Drawing for the job (mm, zero at the part's lowest x, y, z). Coordinates: 2 decimals unless noted, no trailing zeros. Write each loop counter-clockwise with the first axis right and the second up, starting at its lowest first coordinate (ties: lowest second). Pieces come first, ordered by that corner, then holes. Notation, with made-up numbers: M 76.5,29.5 L 108.5,29.5 A17 ccw 108.5,51.5 Z; hole C 18,-19 d4. An arc over 180 degrees is marked long. Put each result on its own line as item: value. Start each with the question number.
Q1. Cut at B-B (z = 5). Write the cut outline in (x, y).
Q2. Cut at D-D (y = 2.75). Write the cut outline in (x, z) (1 decimal).
Q3. Cut at C-C (y = 11.5). Write the cut outline in (x, z).
Q4. Pull direction X, two halves, no side cores. Call the marked faces 1 and 2: pulls with the +X half, pulls with the -X half, needs draft (parallel to the pull), parting line crosses it, or undercut.
Q5. Drill centre lines: line 1 along Z through (x, y) = (8.5, 3.75); line 2 along Y through (x, z) = (7.5, 9) (1 decimal); line 3 along X through (y, z) = (10.25, 3.5). Where is each one in solid material? Low to high.
Q6. Cut at A-A (x = 5). Write the cut outline in (y, z).
Q7. Drop flat-ended pins along their axis: pin 1 (1.5 mm diameter, centred on x = 6.5, y = 2.5, fed in from +Z); pin 2 (3 mm diameter, centred on y = 7, z = 1, fed in from -X); pin 3 (3 mm diameter, centred on x = 8.5, y = 12, fed in from +Z). Give the stop position or say it passes through.
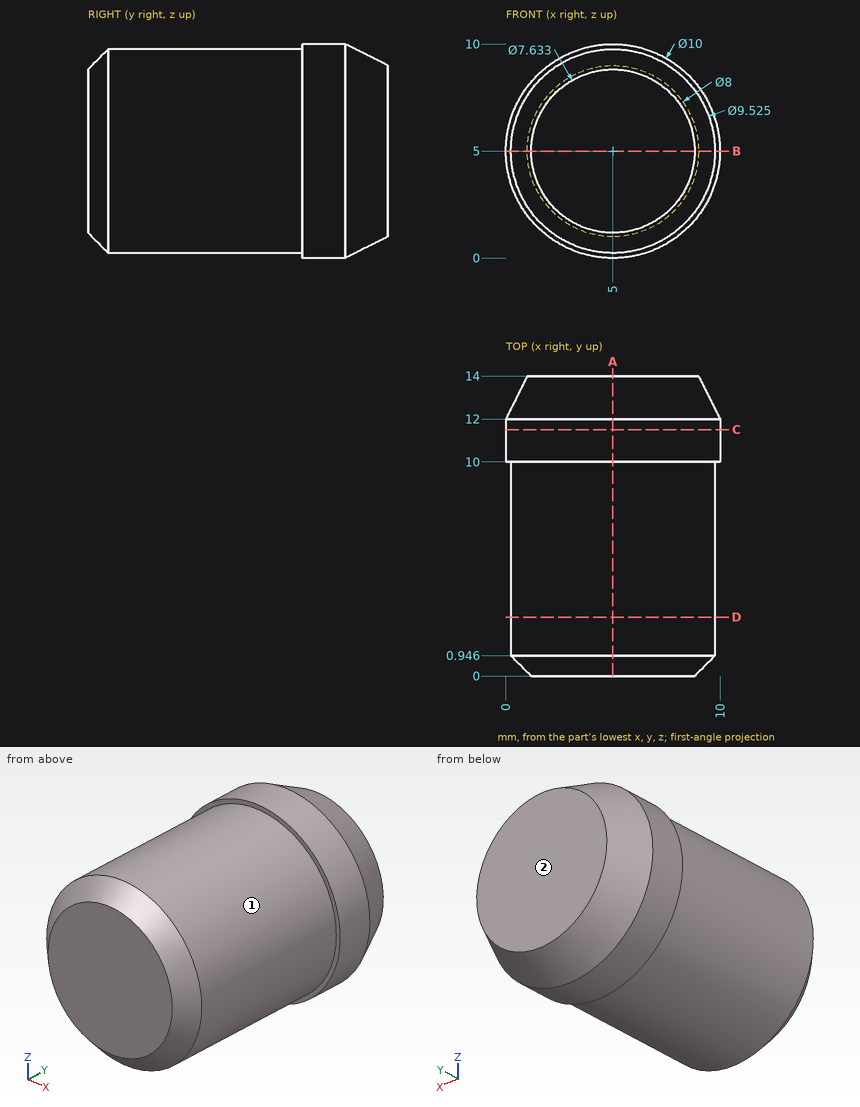
Computed values:
1. outline: M 0,10 L 0.24,10 L 0.24,0.95 L 1.18,0 L 8.82,0 L 9.76,0.95 L 9.76,10 L 10,10 L 10,12 L 9,14 L 1,14 L 0,12 Z
2. outline: C 5,5 d9.5
3. outline: C 5,5 d10
4. face 1: parting line crosses it
4. face 2: needs draft
5. line 1: 1.77 to 8.23
5. line 2: 0.9 to 12.6
5. line 3: 0.23 to 9.77
6. outline: M 0,1.18 L 0.95,0.24 L 10,0.24 L 10,0 L 12,0 L 14,1 L 14,9 L 12,10 L 10,10 L 10,9.76 L 0.95,9.76 L 0,8.82 Z
7. pin 1: z = 9.7
7. pin 2: x = 0.95
7. pin 3: z = 9.58
